Geometry: final body of the model. Coordinates: model frame, mm. A direction names the side the tool comes from. Give positions to 0.01 mm unless a question says otherwise; leave off trailing zeros. Loops run counter-clockwise (first coordinate to the right, second up) from the corner with the lowest first, then second, coordinate; pieces in that order, holes last. Notation, with made-up numbers: (-32, 75.5) -> (-28, 75.5) arc R8 cw to (-28, 81.5) -> close; hole circle Ø4 at (12, 89.25). An arc over 180 degrees is marked (long way). One line per item, written item: value. Start each with the question number.
from build123d import *

# Parameters (mm, degrees)
SKETCH1_W               = 44.45
SKETCH1_H               = 44.45
SKETCH1_W_2             = 38.1
SKETCH1_H_2             = 38.1
BOSS_EXTRUDE1_DEPTH     = 1044.575
F_1_4_CLEARANCE_HOLE3_D = 6.7564
F_1_2_CLEARANCE_HOLE1_D = 13.49248
CUT_EXTRUDE1_DEPTH      = 1046.75651265
SKETCH18_W              = 44.45
SKETCH18_H              = 44.45
SKETCH18_W_2            = 38.1
SKETCH18_H_2            = 38.1
BOSS_EXTRUDE2_DEPTH     = 0.23876


with BuildPart() as part:
    # Sketch1 → Boss-Extrude1 (new body)
    with BuildSketch(Plane.XY):
        Rectangle(SKETCH1_W, SKETCH1_H)
        Rectangle(SKETCH1_W_2, SKETCH1_H_2, mode=Mode.SUBTRACT)
    extrude(amount=BOSS_EXTRUDE1_DEPTH)

    # 1/4 Clearance Hole3 (through all)
    with Locations(Plane(origin=(0, 22.225, 0), x_dir=(1, 0, 0), z_dir=(0, 1, 0))):
        with Locations((0, -318.135), (0, -394.335), (0, -470.535), (0, -788.035), (0, -902.335), (0, -1016.635)):
            Hole(F_1_4_CLEARANCE_HOLE3_D / 2)

    # 1/2 Clearance Hole1 (through all)
    with Locations(Plane(origin=(0, 22.225, 0), x_dir=(1, 0, 0), z_dir=(0, 1, 0))):
        with Locations((0, -260.985)):
            Hole(F_1_2_CLEARANCE_HOLE1_D / 2)

    # Sketch17 → Cut-Extrude1 (cut, through all)
    with BuildSketch(Plane.ZY.offset(22.225)):
        Polygon((282.81376, -22.225), (238.36376, 22.225), (0, 22.225), (0, -22.225), align=None)
    extrude(amount=-CUT_EXTRUDE1_DEPTH, mode=Mode.SUBTRACT)

    # Sketch18 → Boss-Extrude2 (add)
    with BuildSketch(Plane.XY.offset(1044.575)):
        Rectangle(SKETCH18_W, SKETCH18_H)
        Rectangle(SKETCH18_W_2, SKETCH18_H_2, mode=Mode.SUBTRACT)
    extrude(amount=BOSS_EXTRUDE2_DEPTH)


solid = part.part
Item 1: Access query for faces 5 (the face through (-19.05, 0, 638)), 6 (the face through (-22.225, 0, 636)). Directions: +Z, -Z, +X, -X, +Y, -Y. A direction counts if a zero-diameter tool reaches every point of the face in a straight line with its end or side. Return the directions, or none.
Item 2: Section A-A, the plane z = 332. Output: boundary loops of the cut face in (x, y) (3 decimals).
Item 3: Pin query (flat end, axial travel): pin 1 (8 mm diameter, centred on x = 16.5, y = 15, fed in from -Z); pin 2 (3 mm diameter, centred on x = -7.5, y = 18, fed in from -Z). Return the tip coordinate at first contact, or that it passes through.
Item 4: Ray query, line 1 along X through (y, z) = (4.5, 519) (3 decimals); line 2 along Z through (x, y) = (20.5, -1). Return the intervals inside material, ascending. Write a range as [from, to].
Item 5: Section B-B, the plane y = 12. Output: boundary loops of the cut face in (x, z) (3 decimals), then the cut area to 3 significant figures.
Item 6: Mould query, pull axis Y, two halves, no side actions, for faces 1 (the face through (0, 22.225, 636)), 2 (the face through (0, -22.225, 658)), 3 (the face through (19.4, 0.3, 1044.814)), 4 (the face through (0, -19.05, 657)). Classes: pulls with the +Y half, pulls with the -Y half, needs draft (parallel to the pull), parting line crosses it, or undercut.
Geometry check:
1. face 5: +Z, -Z
1. face 6: +Z, -Z, -X, +Y, -Y
2. outline: (-22.225, -22.225) -> (22.225, -22.225) -> (22.225, 22.225) -> (-22.225, 22.225) -> close; hole (-19.05, -19.05) -> (19.05, -19.05) -> (19.05, 19.05) -> (-19.05, 19.05) -> close
3. pin 1: stops at z = 242.51
3. pin 2: stops at z = 241.09
4. line 1: x = [-22.225, -19.05], [19.05, 22.225]
4. line 2: z = [261.59, 1044.81]
5. outline: (-22.225, 248.589) -> (-19.05, 248.589) -> (-19.05, 1044.814) -> (-22.225, 1044.814) -> close; (19.05, 248.589) -> (22.225, 248.589) -> (22.225, 1044.814) -> (19.05, 1044.814) -> close
5. area: 5,060 mm2
6. face 1: pulls with the +Y half
6. face 2: pulls with the -Y half
6. face 3: needs draft
6. face 4: undercut
